from build123d import *

# Parameters (mm, degrees)
SKETCH_1_R          = 12.3
EXTRUDE_1_DEPTH     = 66
SKETCH_2_W          = 15
SKETCH_2_H          = 6
EXTRUDE_2_DEPTH     = 10
SKETCH_3_R          = 3.5
EXTRUDE_3_DEPTH     = 2.5
SKETCH_4_R          = 2
EXTRUDE_4_DEPTH     = 9.5
SKETCH_5_R          = 1.6
CUT_EXTRUDE_1_DEPTH = 4


with BuildPart() as part:
    # 草图1 → 凸台-拉伸1 (new body)
    with BuildSketch(Plane(origin=(0, 0, 0), x_dir=(1, 0, 0), z_dir=(0, 1, 0))):
        with Locations(Location((0, 0, 0), (0, 0, 270))):
            Circle(SKETCH_1_R)
    extrude(amount=EXTRUDE_1_DEPTH)

    # 草图2 → 凸台-拉伸2 (add)
    with BuildSketch(Plane.XY.offset(5)):
        with Locations((0, 57)):
            Rectangle(SKETCH_2_W, SKETCH_2_H)
    extrude(amount=EXTRUDE_2_DEPTH)

    # 草图3 → 凸台-拉伸3 (add)
    with BuildSketch(Plane.XZ):
        with Locations(Location((0, 0, 0), (0, 0, 270))):
            Circle(SKETCH_3_R)
    extrude(amount=EXTRUDE_3_DEPTH)

    # 草图4 → 凸台-拉伸4 (add)
    with BuildSketch(Plane.XZ.offset(2.5)):
        with Locations(Location((0, 0, 0), (0, 0, 270))):
            Circle(SKETCH_4_R)
    extrude(amount=EXTRUDE_4_DEPTH)

    # 草图5 → 切除-拉伸1 (cut)
    with BuildSketch(Plane.XZ):
        with Locations(Location((0, 8.5, 0), (0, 0, 270))):
            Circle(SKETCH_5_R)
        with Locations(Location((0, -8.5, 0), (0, 0, 270))):
            Circle(SKETCH_5_R)
    extrude(amount=-CUT_EXTRUDE_1_DEPTH, mode=Mode.SUBTRACT)


solid = part.part
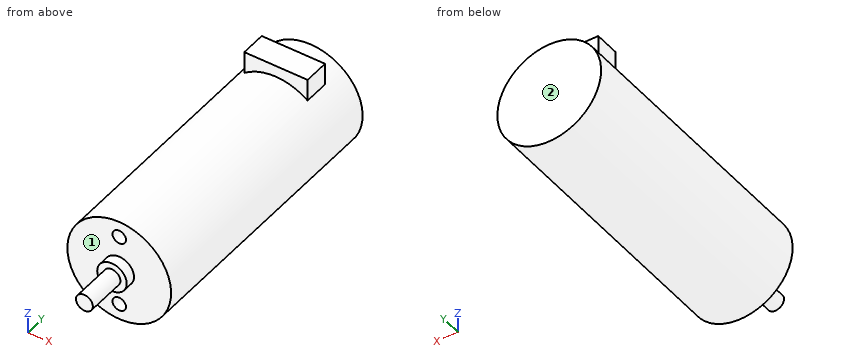
Work out the finished part from the listing and answer in its coordinate system (mm). Face numbers are marked on the shaded views. A direction names the side the tool comes from. Give positions to 0.01 mm unless a question says otherwise; leave off trailing zeros. Write each loop counter-clockwise with the first axis right and the second up, starting at its lowest first coordinate (ties: lowest second). Pieces come first, ordered by that corner, then holes. Notation, with made-up numbers: (42.25, 47) - (65.25, 47) arc R19 cw to (65.25, 58) - close; hole circle Ø11 at (35, 19.25). An arc over 180 degrees is marked (long way). One line per item, written item: value. Start each with the question number.
1. Find section C-C (y = 32). Write down the section's boundary in (x, z).
2. Given pin 1 (3 mm diameter, centred on y = 53.5, z = -9.5, fed in from +X); pin 2 (1 mm diameter, centred on x = 3, y = 21, fed in from +Z); pin 3 (4 mm diameter, centred on x = -9, y = 13.5, fed in from -Z), each flat-ended and moving along its own axis, determine where each tip first touches the part or whether it passes through.
3. Find section D-D (z = 8.5). Write down the section's boundary in (x, y), then the cut area to 3 significant figures.
4. Find section B-B (z = 0). Write down the section's boundary in (x, y).
5. Consider probe 1 along Y at (x, z) = (-6.25, 1); probe 2 along Y at (x, z) = (3.5, 13.5); probe 3 along X at (y, z) = (3, -8.5). Determine where each line is inside the solid, lowest interval first.
6. Find section A-A (x = 0). Write down the section's boundary in (y, z).
7. For the marked faces 1 and 2, determine the directions among +Z, -Z, +X, -X, +Y, -Y from which every point of the face is accessible in a straight line to the end or side of a thin tool.
Geometry results:
1. outline: circle Ø24.6 at (0, 0)
2. pin 1: x = 9.34
2. pin 2: z = 12.04
2. pin 3: z = -10.11
3. outline: (-8.89, 0) - (-1.6, 0) - (-1.6, 4) - (1.6, 4) - (1.6, 0) - (8.89, 0) - (8.89, 66) - (-8.89, 66) - close
3. area: 1,160 mm2
4. outline: (-12.3, 0) - (-3.5, 0) - (-3.5, -2.5) - (-2, -2.5) - (-2, -12) - (2, -12) - (2, -2.5) - (3.5, -2.5) - (3.5, 0) - (12.3, 0) - (12.3, 66) - (-12.3, 66) - close
5. probe 1: 0 to 66
5. probe 2: 54 to 60
5. probe 3: -8.89 to -1.6, 1.6 to 8.89
6. outline: (-12, -2) - (-2.5, -2) - (-2.5, -3.5) - (0, -3.5) - (0, -6.9) - (4, -6.9) - (4, -10.1) - (0, -10.1) - (0, -12.3) - (66, -12.3) - (66, 12.3) - (60, 12.3) - (60, 15) - (54, 15) - (54, 12.3) - (0, 12.3) - (0, 10.1) - (4, 10.1) - (4, 6.9) - (0, 6.9) - (0, 3.5) - (-2.5, 3.5) - (-2.5, 2) - (-12, 2) - close
7. face 1: -Y
7. face 2: +Z, -Z, +X, -X, +Y
